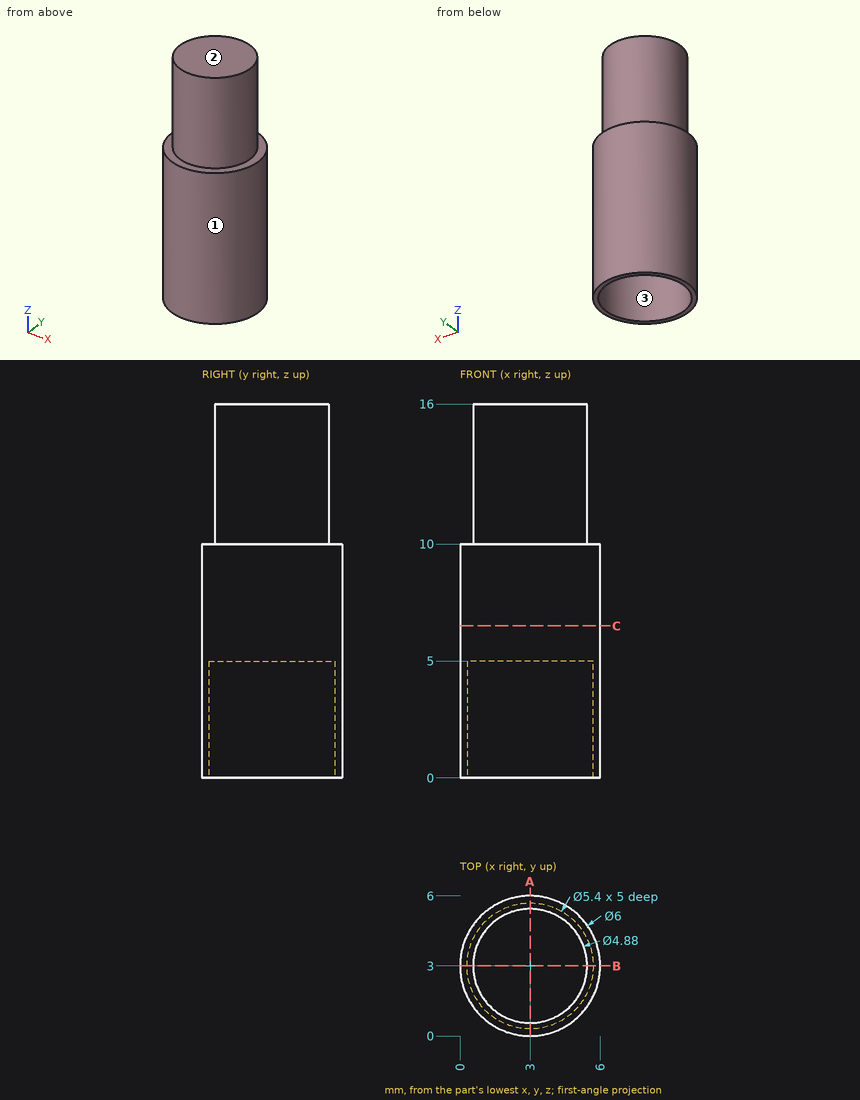
The figure shows three views and two pictorial views of one solid part (mm, origin at its lowest corner). Answer the questions. Round coordinates to 2 decimals unless told otherwise and drop trailing zeros. Order: outer loops, then holes, each group sorted by start corner. A loop starts at its lowest first (then second) coordinate and runs counter-clockwise, first axis right, second up. Notation, with made-up numbers: (67.5, -15) -> (87.5, -15) arc R16 ccw to (87.5, 12) -> close; hole circle Ø6 at (79, 89). An arc over 180 degrees is marked (long way). Put each result on its own line as item: value.
Q1. Section A-A, the plane x = 3 is taken. Write down the section's boundary in (y, z).
Results list:
outline: (0, 0) -> (0.3, 0) -> (0.3, 5) -> (5.7, 5) -> (5.7, 0) -> (6, 0) -> (6, 10) -> (5.44, 10) -> (5.44, 16) -> (0.56, 16) -> (0.56, 10) -> (0, 10) -> close
Q2. Consider line 1 along Y through (x, z) = (3, 1.25); line 2 along Z through (x, y) = (3.75, 1.15); line 3 along Z through (x, y) = (4.35, 5.5). Determine where each line is inside the solid, lowest interval first.
Results list:
line 1: 0 to 0.3, 5.7 to 6
line 2: 5 to 16
line 3: 0 to 10
Q3. Determine the mould class of the marked faces 1, 2 and 3 for opening direction Y: pulls with the +Y half, pulls with the -Y half, needs draft (parallel to the pull), parting line crosses it, or undercut.
Results list:
face 1: parting line crosses it
face 2: needs draft
face 3: undercut
Q4. Section C-C, the plane z = 6.5 is taken. Write down the section's boundary in (x, y).
Results list:
outline: circle Ø6 at (3, 3)
